CAD build for the part. Positions are in the model's coordinates, mm. A direction names the side the tool comes from. Round coordinates to 2 decimals unless told otherwise and drop trailing zeros. Write each loop counter-clockwise with the first axis right and the second up, starting at its lowest first coordinate (ties: lowest second). Pieces come first, ordered by that corner, then holes. Notation, with made-up numbers: (41, 30.25) -> (48, 30.25) arc R30 ccw to (48, 59.25) -> close; hole circle Ø1 at (38, 83). An arc over 180 degrees is marked (long way). Put each result on its own line as item: value. Start each with the question number.
1. Drill centre lines: line 1 (Y direction, x = -8.5, z = 1.75); line 2 (Y direction, x = 11.5, z = 2.05); line 3 (X direction, y = -4, z = 0.3). Where is each one in solid material? Low to high. Write a range as from..to.
2. Pull direction X, two halves, no side cores. Call faces 3 (the flat face through (-74.243, 44.613, 1.479)), 4 (the flat face through (-2, 29, 0)), 5 (the flat face through (75.757, 41.989, 1.479)), 6 (the flat face through (-37.649, 58.275, 1.479)): pulls with the +X half, pulls with the -X half, needs draft (parallel to the pull), parting line crosses it, or undercut.
3. 3-axis set-ups, long thin cutter, end or side, ignore diameter. For faces 1 (the flat face through (-2, 29, 3)), 2 (the flat face through (-53.518, 10.51, 1.479)): which of +Z, -Z, +X, -X, +Y, -Y reach the whole face in a straight line?
4. Saw through at A-A on x = -62.5. List the corners of the cut face in (y, z).
5. Saw through at B-B on y = 8. List the corners of the cut face in (x, z), and give its area (3 significant figures).
6. Saw through at C-C on x = 55.5. List the corners of the cut face in (y, z).
7. Flat gauge pins, fed straight in: P1, Ø1.9, axis at x = 106.82, y = -78.99, coming from the -Z side; P2, Ø1.5, axis at y = -46.5, z = 1, coming from the -X side. Where does each tip first touch, or does it go through?
8. Saw through at D-D on z = 2.4. State how many separate pieces and enclosed holes the cut face has, and give its area (3 significant figures).
from build123d import *

# Parameters (mm, degrees)
SKETCH_1_R      = 1.6
SKETCH_1_R_2    = 1.1
SKETCH_1_W      = 48
SKETCH_1_H      = 38
SKETCH_1_W_2    = 70
SKETCH_1_H_2    = 41.397849463
EXTRUDE_1_DEPTH = 3
FILLET_1_R      = 10


with BuildPart() as part:
    # 草图1 → 凸台-拉伸1 (new body)
    with BuildSketch(Plane.XY):
        Polygon((-18.016261775, 142), (-131.983738225, -55.397459622), (-113.96747645, -86.602540378), (113.96747645, -86.602540378), (131.983738225, -55.397459622), (18.016261775, 142), align=None)
        with Locations((-15, 132)):
            Circle(SKETCH_1_R, mode=Mode.SUBTRACT)
        with Locations((15, 132)):
            Circle(SKETCH_1_R, mode=Mode.SUBTRACT)
        with Locations((15, 108)):
            Circle(SKETCH_1_R, mode=Mode.SUBTRACT)
        with Locations((-15, 108)):
            Circle(SKETCH_1_R, mode=Mode.SUBTRACT)
        with Locations((-29, 24)):
            Circle(SKETCH_1_R, mode=Mode.SUBTRACT)
        with Locations((-29, -24)):
            Circle(SKETCH_1_R, mode=Mode.SUBTRACT)
        with Locations((-86.030743609, -66.990381057)):
            Circle(SKETCH_1_R, mode=Mode.SUBTRACT)
        with Locations((29, -24)):
            Circle(SKETCH_1_R, mode=Mode.SUBTRACT)
        with Locations((29, 24)):
            Circle(SKETCH_1_R, mode=Mode.SUBTRACT)
        with Locations((101.030743609, -41.009618943)):
            Circle(SKETCH_1_R, mode=Mode.SUBTRACT)
        with Locations((86.030743609, -66.990381057)):
            Circle(SKETCH_1_R, mode=Mode.SUBTRACT)
        with Locations((106.8153533, -78.990381057)):
            Circle(SKETCH_1_R, mode=Mode.SUBTRACT)
        with Locations((121.8153533, -53.009618943)):
            Circle(SKETCH_1_R, mode=Mode.SUBTRACT)
        with Locations((-101.030743609, -41.009618943)):
            Circle(SKETCH_1_R, mode=Mode.SUBTRACT)
        with Locations((-121.8153533, -53.009618943)):
            Circle(SKETCH_1_R, mode=Mode.SUBTRACT)
        with Locations((-106.8153533, -78.990381057)):
            Circle(SKETCH_1_R, mode=Mode.SUBTRACT)
        with Locations((-11.5, 84)):
            Circle(SKETCH_1_R_2, mode=Mode.SUBTRACT)
        with Locations((11.5, 84)):
            Circle(SKETCH_1_R_2, mode=Mode.SUBTRACT)
        with Locations((11.5, 59)):
            Circle(SKETCH_1_R_2, mode=Mode.SUBTRACT)
        with Locations((-11.5, 59)):
            Circle(SKETCH_1_R_2, mode=Mode.SUBTRACT)
        with Locations((-46.5, -27.602540378)):
            Circle(SKETCH_1_R, mode=Mode.SUBTRACT)
        with Locations((-46.5, -82.602540378)):
            Circle(SKETCH_1_R, mode=Mode.SUBTRACT)
        with Locations((46.5, -82.602540378)):
            Circle(SKETCH_1_R, mode=Mode.SUBTRACT)
        with Locations((46.5, -27.602540378)):
            Circle(SKETCH_1_R, mode=Mode.SUBTRACT)
        Rectangle(SKETCH_1_W, SKETCH_1_H, mode=Mode.SUBTRACT)
        Polygon((-46.188021535, 63.205080757), (-28.867513459, 53.205080757), (-78.867513459, -33.397459622), (-96.188021535, -23.397459622), align=None, mode=Mode.SUBTRACT)
        with Locations((0, -55.102540379)):
            Rectangle(SKETCH_1_W_2, SKETCH_1_H_2, mode=Mode.SUBTRACT)
        Polygon((46.188021535, 63.205080757), (28.867513459, 53.205080757), (78.867513459, -33.397459622), (96.188021535, -23.397459622), align=None, mode=Mode.SUBTRACT)
    extrude(amount=EXTRUDE_1_DEPTH)

    # 圆角1
    fillet_1_edges = [part.edges().sort_by_distance(p)[0] for p in [
        (-131.983738225, -55.397459622, 1.5),
        (-18.016261775, 142, 1.5),
        (18.016261775, 142, 1.5),
        (131.983738225, -55.397459622, 1.5),
        (113.96747645, -86.602540378, 1.5),
        (-113.96747645, -86.602540378, 1.5),
    ]]
    fillet(fillet_1_edges, radius=FILLET_1_R)


solid = part.part
Return value:
1. line 1: y = -86.6..-75.8, -34.4..-19, 19..142
1. line 2: y = -86.6..-75.8, -34.4..-19, 19..57.9, 60.1..82.9, 85.1..142
1. line 3: x = -102.31..-84.99, -61.89..-24, 24..61.89, 84.99..102.31
2. face 3: pulls with the -X half
2. face 4: needs draft
2. face 5: pulls with the +X half
2. face 6: undercut
3. face 1: +Z, +X, -X, +Y, -Y
3. face 2: +Z, -Z
4. outline: (-86.6, 0) -> (-5.05, 0) -> (-5.05, 3) -> (-86.6, 3) -> close; (34.95, 0) -> (64.95, 0) -> (64.95, 3) -> (34.95, 3) -> close
5. outline: (-95.38, 0) -> (-78.06, 0) -> (-78.06, 3) -> (-95.38, 3) -> close; (-54.97, 0) -> (-24, 0) -> (-24, 3) -> (-54.97, 3) -> close; (24, 0) -> (54.97, 0) -> (54.97, 3) -> (24, 3) -> close; (78.06, 0) -> (95.38, 0) -> (95.38, 3) -> (78.06, 3) -> close
5. area: 290 mm^2
6. outline: (-86.6, 0) -> (7.08, 0) -> (7.08, 3) -> (-86.6, 3) -> close; (47.08, 0) -> (77.08, 0) -> (77.08, 3) -> (47.08, 3) -> close
7. P1: passes through
7. P2: stops at x = -127.28
8. separate pieces: 1
8. enclosed holes: 28
8. area: 28,400 mm^2
